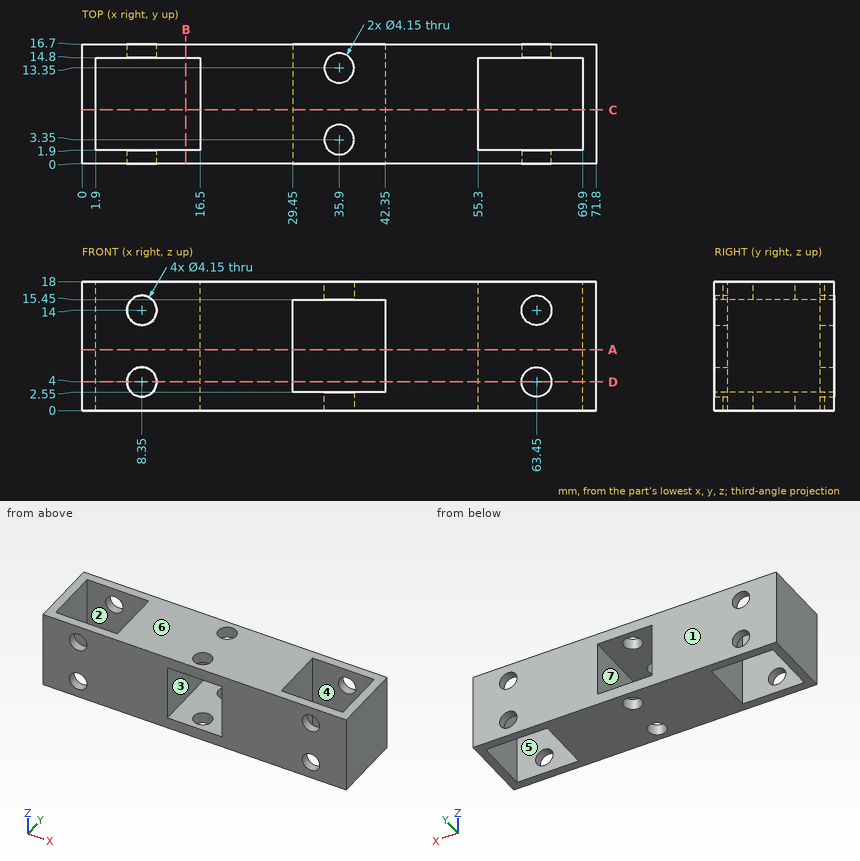
For this review, use the dimensioned drawing (mm, ordinates from the lowest corner) and the shaded views. A direction names the side the tool comes from. Round coordinates to 2 decimals unless told otherwise and drop trailing zeros. Order: outer loops, then holes, each group sorted by start corner. A loop starts at its lowest first (then second) coordinate and runs counter-clockwise, first axis right, second up. Notation, with made-up numbers: (28, -35) - (44, -35) arc R22 ccw to (44, -25) - close; hole circle Ø2 at (8, 48.5). An arc over 180 degrees is marked (long way). Use one line per item in the form item = value.
Q1. To check wall thickness, follow line 1 (Y direction, x = 35.9, z = 1.75) (3 decimals); line 2 (X direction, y = 2.25, z = 10.5); line 3 (Z direction, x = 8.35, y = 0.8) (3 decimals). State the ranges of each line that lie inside material, in increasing order.
Response values:
line_1 = 0 to 1.275, 5.425 to 11.275, 15.425 to 16.7
line_2 = 0 to 1.9, 16.5 to 29.45, 42.35 to 55.3, 69.9 to 71.8
line_3 = 0 to 1.925, 6.075 to 11.925, 16.075 to 18
Q2. Tool access review of the marked faces 5, 6 and 7: name each direction out of +Z, -Z, +X, -X, +Y, -Y from which nothing blocks a thin tool from reaching the whole face with its end or side.
Response values:
face_5 = +Z, -Z
face_6 = +Z, +X, -X, +Y, -Y
face_7 = +Y, -Y
Q3. Add section D-D on z = 4. Give the number of separate pieces and of enclosed holes in the cut face, then the cut area to 3 significant figures.
Response values:
separate_pieces = 4
enclosed_holes = 0
area = 575 mm^2
Q4. Mouldability with a two-part tool opening along Y and no side actions: class the marked faces 1, 2, 3 and 4 as pulls with the +Y half, pulls with the -Y half, needs draft (parallel to the pull), parting line crosses it, or undercut.
Response values:
face_1 = pulls with the +Y half
face_2 = undercut
face_3 = needs draft
face_4 = undercut
Q5. Add section B-B on x = 14.5. Give the boundary of the cut face in (y, z), then the cut area to 3 significant figures.
Response values:
outline = (0, 0) - (1.9, 0) - (1.9, 18) - (0, 18) - close; (14.8, 0) - (16.7, 0) - (16.7, 18) - (14.8, 18) - close
area = 68.4 mm^2
Q6. Add section A-A on z = 8.5. Give the boundary of the cut face in (x, y).
Response values:
outline = (0, 0) - (29.45, 0) - (29.45, 16.7) - (0, 16.7) - close; (42.35, 0) - (71.8, 0) - (71.8, 16.7) - (42.35, 16.7) - close; hole (1.9, 1.9) - (16.5, 1.9) - (16.5, 14.8) - (1.9, 14.8) - close; hole (55.3, 1.9) - (69.9, 1.9) - (69.9, 14.8) - (55.3, 14.8) - close
Q7. Add section C-C on y = 7.5. Give the boundary of the cut face in (x, z), then the cut area to 3 significant figures.
Response values:
outline = (0, 0) - (1.9, 0) - (1.9, 18) - (0, 18) - close; (16.5, 0) - (55.3, 0) - (55.3, 18) - (16.5, 18) - close; (69.9, 0) - (71.8, 0) - (71.8, 18) - (69.9, 18) - close; hole (29.45, 2.55) - (42.35, 2.55) - (42.35, 15.45) - (29.45, 15.45) - close
area = 600 mm^2
